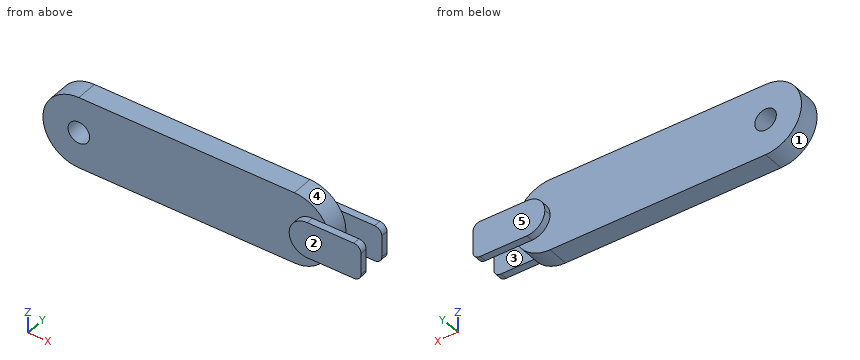
from build123d import *

# Parameters (mm, degrees)
BOSS_EXTRUDE1_DEPTH = 3
SKETCH5_W           = 10
SKETCH5_H           = 1
BOSS_EXTRUDE2_DEPTH = 2.5
FILLET1_R           = 2.5
FILLET2_R           = 1
SKETCH6_R           = 1.5
CUT_EXTRUDE1_DEPTH  = 41.509258201


with BuildPart() as part:
    # Sketch2 → Boss-Extrude1 (new body)
    with BuildSketch(Plane(origin=(0, 0, 0), x_dir=(1, 0, 0), z_dir=(0, 1, 0))):
        with BuildLine():
            Line((0, 5), (30, 5))
            ThreePointArc((30, 5), (35, 0), (30, -5))
            Line((30, -5), (0, -5))
            ThreePointArc((0, -5), (-5, 0), (0, 5))
        make_face()
    extrude(amount=BOSS_EXTRUDE1_DEPTH)

    # Sketch5 → Boss-Extrude2 (add, symmetric)
    with BuildSketch(Plane.XY):
        with Locations((35, 3.5)):
            Rectangle(SKETCH5_W, SKETCH5_H)
        with Locations((35, -0.5)):
            Rectangle(SKETCH5_W, SKETCH5_H)
    extrude(amount=BOSS_EXTRUDE2_DEPTH, both=True)

    # Fillet1
    fillet1_edges = [part.edges().sort_by_distance(p)[0] for p in [
        (30, -0.5, 2.5),
        (30, -0.5, -2.5),
        (30, 3.5, -2.5),
        (30, 3.5, 2.5),
    ]]
    fillet(fillet1_edges, radius=FILLET1_R - 0.0001)  # a hair under: the kernel refuses the full size

    # Fillet2
    fillet2_edges = [part.edges().sort_by_distance(p)[0] for p in [
        (40, 3.5, -2.5),
        (40, 3.5, 2.5),
        (40, -0.5, -2.5),
        (40, -0.5, 2.5),
    ]]
    fillet(fillet2_edges, radius=FILLET2_R)

    # Sketch6 → Cut-Extrude1 (cut, through all)
    with BuildSketch(Plane(origin=(0, 3, 0), x_dir=(1, 0, 0), z_dir=(0, 1, 0))):
        with Locations(Location((0, 0, 0), (0, 0, 270))):
            Circle(SKETCH6_R)
    extrude(amount=-CUT_EXTRUDE1_DEPTH, mode=Mode.SUBTRACT)


solid = part.part
Input: part model. Units: mm. Frame: model coordinates. Face numbers are marked on the shaded views. A direction names the side the tool comes from. Give positions to 0.01 mm unless a question says otherwise; leave off trailing zeros. Loops run counter-clockwise (first coordinate to the right, second up) from the corner with the lowest first, then second, coordinate; pieces in that order, holes last. Notation, with made-up numbers: (3.5, 37) -> (15.5, 37) arc R9 cw to (15.5, 42) -> close; hole circle Ø1 at (-1, 3.5). An arc over 180 degrees is marked (long way). Answer as a JSON object with one key per item and string values. Group by question number.
Item 1: Cut plane B-B, the plane x = 15.5. Return the cut outline in (y, z).
Item 2: Pin query (flat end, axial travel): P1, Ø0.8, axis at x = 34.5, y = 3.5, coming from the -Z side; P2, Ø4, axis at x = 14.5, z = -1, coming from the -Y side; P3, Ø0.5, axis at x = 35, y = 3.5, coming from the +Z side. Return the tip coordinate at first contact, or that it passes through.
Item 3: Line query: probe 1 along X at (y, z) = (1.15, 0); probe 2 along Y at (x, z) = (19, -3); probe 3 along X at (y, z) = (1.7, 1.25). Output: solid intervals per line, ascending.
Item 4: Reachability of the marked faces 4 and 5 from +Z, -Z, +X, -X, +Y, -Y: full face, straight path, thin tool, end or side. Return the list, or none.
Item 5: Cut plane C-C, the plane z = 4. Return the cut outline in (x, y).
Item 6: Cut plane A-A, the plane y = 2.3. Return the cut outline in (x, z).
Item 7: Pull-direction query (Y, two-part tool) for the marked faces 1, 2 and 3; classes: released by +Y, released by -Y, zero draft, split by the parting line, or undercut.
Checks:
{
 "1": {"outline": "(0, -5) -> (3, -5) -> (3, 5) -> (0, 5) -> close"},
 "2": {"P1": "stops at z = -2.5", "P2": "stops at y = 0", "P3": "stops at z = 2.5"},
 "3": {"probe 1": "x = -5 to -1.5, 1.5 to 35", "probe 2": "y = 0 to 3", "probe 3": "x = -4.84 to -0.83, 0.83 to 34.84"},
 "4": {"face 4": "+X", "face 5": "+Z, -Z, +X, -X, +Y"},
 "5": {"outline": "(-3, 0) -> (33, 0) -> (33, 3) -> (-3, 3) -> close"},
 "6": {"outline": "(0, -5) -> (30, -5) arc R5 ccw to (30, 5) -> (0, 5) arc R5 ccw to start; hole circle Ø3 at (0, 0)"},
 "7": {"face 1": "zero draft", "face 2": "released by -Y", "face 3": "undercut"}
}
